Here's how the part is built. I have some questions about the finished solid (model axes, mm). A direction names the side the tool comes from. Coordinates: 2 decimals unless noted, no trailing zeros. Write each loop counter-clockwise with the first axis right and the second up, starting at its lowest first coordinate (ties: lowest second). Pieces come first, ordered by that corner, then holes. Notation, with made-up numbers: (-12, 45) -> (16, 45) arc R33 ccw to (16, 73) -> close; hole circle Ø4 at (-22, 62). An arc over 180 degrees is marked (long way). Put each result on its own line as item: value.
```python
from build123d import *

# Parameters (mm, degrees)
SKETCH1_W           = 75
SKETCH1_H           = 75
SKETCH1_R           = 3.3
SKETCH1_R_2         = 1.1303
BOSS_EXTRUDE1_DEPTH = 12.7
SKETCH2_R           = 5.1
CUT_EXTRUDE1_DEPTH  = 4
CUT_EXTRUDE2_DEPTH  = 1.8


with BuildPart() as part:
    # Sketch1 → Boss-Extrude1 (new body)
    with BuildSketch(Plane.XY):
        with Locations((-35.66615728, 23.529473029)):
            Rectangle(SKETCH1_W, SKETCH1_H)
        with Locations((-60.66615728, -1.470526971)):
            Circle(SKETCH1_R, mode=Mode.SUBTRACT)
        with Locations((-10.66615728, -1.470526971)):
            Circle(SKETCH1_R, mode=Mode.SUBTRACT)
        with Locations((-10.66615728, 48.529473029)):
            Circle(SKETCH1_R, mode=Mode.SUBTRACT)
        with Locations((-60.66615728, 48.529473029)):
            Circle(SKETCH1_R, mode=Mode.SUBTRACT)
        with Locations((-60.66615728, 33.529473029)):
            Circle(SKETCH1_R_2, mode=Mode.SUBTRACT)
        with Locations((-10.66615728, 33.529473029)):
            Circle(SKETCH1_R_2, mode=Mode.SUBTRACT)
        with Locations((-60.66615728, 13.529473029)):
            Circle(SKETCH1_R_2, mode=Mode.SUBTRACT)
        with Locations((-10.66615728, 13.529473029)):
            Circle(SKETCH1_R_2, mode=Mode.SUBTRACT)
    extrude(amount=BOSS_EXTRUDE1_DEPTH)

    # Sketch2 → Cut-Extrude1 (cut)
    with BuildSketch(Plane.XY.offset(12.7)):
        with Locations((-60.66615728, 48.529473029)):
            Circle(SKETCH2_R)
        with Locations((-10.66615728, 48.529473029)):
            Circle(SKETCH2_R)
        with Locations((-60.66615728, -1.470526971)):
            Circle(SKETCH2_R)
        with Locations((-10.66615728, -1.470526971)):
            Circle(SKETCH2_R)
    extrude(amount=-CUT_EXTRUDE1_DEPTH, mode=Mode.SUBTRACT)

    # Sketch3 → Cut-Extrude2 (cut)
    with BuildSketch(Plane.XY.offset(12.7)):
        with BuildLine():
            Line((-49.663826945, 39.194037394), (-25.013826945, 39.194037394))
            Line((-25.013826945, 39.194037394), (-25.013826945, 61.029473029))
            Line((-25.013826945, 61.029473029), (-21.838826945, 61.029473029))
            Line((-21.838826945, 61.029473029), (-21.838826945, 39.194037394))
            Line((-21.838826945, 39.194037394), (-21.838826945, 9.781537394))
            ThreePointArc((-21.838826945, 9.781537394), (-20.71629493, 7.071505379), (-23.426326945, 8.194037394))
            Line((-23.426326945, 8.194037394), (-51.251326945, 8.194037394))
            ThreePointArc((-51.251326945, 8.194037394), (-53.96135896, 7.071505379), (-52.838826945, 9.781537394))
            Line((-52.838826945, 9.781537394), (-52.838826945, 39.194037394))
            Line((-52.838826945, 39.194037394), (-52.838826945, 61.029473029))
            Line((-52.838826945, 61.029473029), (-49.663826945, 61.029473029))
            Line((-49.663826945, 61.029473029), (-49.663826945, 39.194037394))
        make_face()
    extrude(amount=-CUT_EXTRUDE2_DEPTH, mode=Mode.SUBTRACT)


solid = part.part
```
Item 1: Please list where these lines run through material, in increasing order: line 1 along Y through (x, z) = (-59.5, 2.75); line 2 along Y through (x, z) = (-42, 12.25); line 3 along X through (y, z) = (0.5, 3.5). Write a range as from..to.
Output:
line 1: y = -13.97..-4.56, 1.62..45.44, 51.62..61.03
line 2: y = -13.97..8.19, 39.19..61.03
line 3: x = -73.17..-63.31, -58.02..-13.31, -8.02..1.83
Item 2: Imagine slicing it at A-A on y = 31.5. Write out the boundary of the cut face in (x, z).
Output:
outline: (-73.17, 0) -> (1.83, 0) -> (1.83, 12.7) -> (-21.84, 12.7) -> (-21.84, 10.9) -> (-52.84, 10.9) -> (-52.84, 12.7) -> (-73.17, 12.7) -> close
Item 3: If we mould it in two halves opening along X, with no side actions, what happens to faces 1 (the flat face through (-36, 24, 0)), 2 (the flat face through (1.834, 23, 6)), 3 (the flat face through (-52.839, 35, 12)), 4 (the flat face through (-37, 28, 10.9))? For each: released by +X, released by -X, zero draft, split by the parting line, or undercut.
Output:
face 1: zero draft
face 2: released by +X
face 3: undercut
face 4: undercut
Item 4: For P1, Ø8.5, axis at x = -60.67, y = 48.53, coming from the +Z side, with a flat end and sliding along its axis, tell me the tip position at first contact or that it passes through.
Output:
P1: stops at z = 8.7
Item 5: Imagine slicing it at B-B on x = -31. Write out the boundary of the cut face in (y, z), then the cut area to 3 significant figures.
Output:
outline: (-13.97, 0) -> (61.03, 0) -> (61.03, 12.7) -> (39.19, 12.7) -> (39.19, 10.9) -> (8.19, 10.9) -> (8.19, 12.7) -> (-13.97, 12.7) -> close
area: 897 mm²
Item 6: Which directions (+Z, -Z, +X, -X, +Y, -Y) give clear straight access to the entire face, cutting with the end or side of a thin tool? Please do faces 5 (the flat face through (-7, 49, 8.7)), 6 (the cylindrical face through (-11.382, 45.308, 4.289)), 7 (the flat face through (-21.839, 36, 12)).
Output:
face 5: +Z
face 6: +Z, -Z
face 7: +Z, +Y
Item 7: Imagine slicing it at C-C on z = 5. State how many separate pieces and enclosed holes the cut face has, then the cut area to 3 significant figures.
Output:
separate pieces: 1
enclosed holes: 8
area: 5,470 mm²
